from build123d import *

# Parameters (mm, degrees)
ESQUISSE1_R             = 22.5
BOSS_EXTRU_1_DEPTH      = 3
ESQUISSE2_R             = 5
BOSS_EXTRU_2_DEPTH      = 3
ENL_V_MAT_EXTRU_3_DEPTH = 10
ESQUISSE10_R            = 1.5
ENL_V_MAT_EXTRU_4_DEPTH = 10
ENL_V_MAT_EXTRU_5_DEPTH = 2.1
ESQUISSE12_R            = 0.515
ESQUISSE12_R_2          = 1.235
ENL_V_MAT_EXTRU_6_DEPTH = 33.057916339
ESQUISSE13_R            = 1.5
ENL_V_MAT_EXTRU_7_DEPTH = 33.380549717


with BuildPart() as part:
    # Esquisse1 → Boss.-Extru.1 (new body)
    with BuildSketch(Plane.XY):
        Circle(ESQUISSE1_R)
    extrude(amount=BOSS_EXTRU_1_DEPTH)

    # Esquisse2 → Boss.-Extru.2 (add)
    with BuildSketch(Plane.XY.offset(3)):
        Circle(ESQUISSE2_R)
    extrude(amount=BOSS_EXTRU_2_DEPTH)

    # Esquisse6 → Enlèv. mat.-Extru.3 (cut)
    with BuildSketch(Plane(origin=(0, 0, 0), x_dir=(-1, 0, 0), z_dir=(0, 0, -1))):
        with BuildLine():
            Line((-5, 19), (5, 19))
            ThreePointArc((5, 19), (6, 18), (5, 17))
            Line((5, 17), (-5, 17))
            ThreePointArc((-5, 17), (-6, 18), (-5, 19))
        make_face()
    extrude(amount=-ENL_V_MAT_EXTRU_3_DEPTH, mode=Mode.SUBTRACT)

    # Esquisse10 → Enlèv. mat.-Extru.4 (cut)
    with BuildSketch(Plane(origin=(0, 0, 0), x_dir=(-1, 0, 0), z_dir=(0, 0, -1))):
        with Locations((-9.835, -12)):
            Circle(ESQUISSE10_R)
        with Locations((9.831247904, -12)):
            Circle(ESQUISSE10_R)
    extrude(amount=-ENL_V_MAT_EXTRU_4_DEPTH, mode=Mode.SUBTRACT)

    # Esquisse11 → Enlèv. mat.-Extru.5 (cut)
    with BuildSketch(Plane.XY.offset(6)):
        with BuildLine():
            Line((2.516635816, 4.378246701), (2.643897714, 2.262786971))
            ThreePointArc((2.643897714, 2.262786971), (3.48, 0), (2.643897714, -2.262786971))
            Line((2.643897714, -2.262786971), (2.516635816, -4.378246701))
            ThreePointArc((2.516635816, -4.378246701), (0, -5.05), (-2.516635816, -4.378246701))
            Line((-2.516635816, -4.378246701), (-2.643897714, -2.262786971))
            ThreePointArc((-2.643897714, -2.262786971), (-3.48, 0), (-2.643897714, 2.262786971))
            Line((-2.643897714, 2.262786971), (-2.516635816, 4.378246701))
            ThreePointArc((-2.516635816, 4.378246701), (0, 5.05), (2.516635816, 4.378246701))
        make_face()
    extrude(amount=-ENL_V_MAT_EXTRU_5_DEPTH, mode=Mode.SUBTRACT)

    # Esquisse12 → Enlèv. mat.-Extru.6 (cut, through all)
    with BuildSketch(Plane.XY.offset(3.9)):
        with Locations((0, 4.25)):
            Circle(ESQUISSE12_R)
        Circle(ESQUISSE12_R_2)
        with Locations((0, -4.25)):
            Circle(ESQUISSE12_R)
    extrude(amount=-ENL_V_MAT_EXTRU_6_DEPTH, mode=Mode.SUBTRACT)

    # Esquisse13 → Enlèv. mat.-Extru.7 (cut, through all)
    with BuildSketch(Plane(origin=(0, 0, 0), x_dir=(-1, 0, 0), z_dir=(0, 0, -1))):
        with Locations((-9.835, 15.615)):
            Circle(ESQUISSE13_R)
        with Locations((9.831247904, 15.615)):
            Circle(ESQUISSE13_R)
    extrude(amount=-ENL_V_MAT_EXTRU_7_DEPTH, mode=Mode.SUBTRACT)


solid = part.part
Model file for the job. Use its own axes, mm. A direction names the side the tool comes from. Coordinates: 2 decimals unless noted, no trailing zeros. Loops run counter-clockwise (first coordinate to the right, second up) from the corner with the lowest first, then second, coordinate; pieces in that order, holes last. Notation, with made-up numbers: (6, -36) -> (41, -36) arc R16 ccw to (41, -6) -> close; hole circle Ø2 at (5, 75.25). An arc over 180 degrees is marked (long way). Use one line per item in the form item = value. Start each with the question number.
(1) Flat gauge pins, fed straight in: pin 1 (2 mm diameter, centred on x = -10, y = -2.5, fed in from +Z); pin 2 (1.5 mm diameter, centred on x = 2, z = 2, fed in from -Y); pin 3 (2.5 mm diameter, centred on x = 9.835, y = -12, fed in from +Z); pin 4 (1.6 mm diameter, centred on x = 0, y = -4.25, fed in from +Z). Where does each tip first touch, or does it go through?
(2) Cut at B-B on y = 0. Give the cut face in (x, z) (3 decimals).
(3) Cut at C-C on z = 1.8. Give the number of separate pieces and of enclosed holes in the cut face, and give its area (3 significant figures).
(4) Tool access for faces 1 (the flat face through (-4, 0, 6)), 2 (the flat face through (0, 19, 1)), 3 (the flat face through (2.583, -3.276, 4.965)): list every direction of +Z, -Z, +X, -X, +Y, -Y with a clear straight run to the whole face (end or side of a thin tool).
(5) Pull direction Y, two halves, no side cores. Call faces 4 (the flat face through (2.58, 3.3, 4.96)), 5 (the flat face through (0, -5, 0)), 6 (the cylindrical face through (-0.651, 4.957, 3.479)): pulls with the +Y half, pulls with the -Y half, needs draft (parallel to the pull), parting line crosses it, or undercut.
(6) Cut at D-D on y = -12. Give the cut face in (x, z) (3 decimals).
(7) Probe probe 1 along Y at (x, z) = (0, 2.2) (3 decimals); probe 2 along Z at (x, y) = (7, 17); probe 3 along X at (y, z) = (-4.5, 1.2). List the from-to ranges inside material, lowest first. Write a range as from..to.
(8) Cut at A-A on x = 0. Give the cut face in (y, z) (3 decimals), and give its area (3 significant figures).
Values:
q1.pin_1 = 3
q1.pin_2 = -22.47
q1.pin_3 = through
q1.pin_4 = 3.9
q2.outline = (-22.5, 0) -> (-1.235, 0) -> (-1.235, 3.9) -> (-3.48, 3.9) -> (-3.48, 6) -> (-5, 6) -> (-5, 3) -> (-22.5, 3) -> close; (1.235, 0) -> (22.5, 0) -> (22.5, 3) -> (5, 3) -> (5, 6) -> (3.48, 6) -> (3.48, 3.9) -> (1.235, 3.9) -> close
q3.separate_pieces = 1
q3.enclosed_holes = 8
q3.area = 1,530 mm2
q4.face_1 = +Z, +X, -X, +Y, -Y
q4.face_2 = +Z, -Z
q4.face_3 = +Z
q5.face_4 = undercut
q5.face_5 = needs draft
q5.face_6 = parting line crosses it
q6.outline = (-19.033, 0) -> (-11.331, 0) -> (-11.331, 3) -> (-19.033, 3) -> close; (-8.331, 0) -> (8.335, 0) -> (8.335, 3) -> (-8.331, 3) -> close; (11.335, 0) -> (19.033, 0) -> (19.033, 3) -> (11.335, 3) -> close
q7.probe_1 = -22.5..-4.765, -3.735..-1.235, 1.235..3.735, 4.765..17, 19..22.5
q7.probe_2 = 0..3
q7.probe_3 = -22.05..-0.45, 0.45..22.05
q8.outline = (-22.5, 0) -> (-4.765, 0) -> (-4.765, 3.9) -> (-5, 3.9) -> (-5, 3) -> (-22.5, 3) -> close; (-3.735, 0) -> (-1.235, 0) -> (-1.235, 3.9) -> (-3.735, 3.9) -> close; (1.235, 0) -> (3.735, 0) -> (3.735, 3.9) -> (1.235, 3.9) -> close; (4.765, 0) -> (17, 0) -> (17, 3) -> (5, 3) -> (5, 3.9) -> (4.765, 3.9) -> close; (19, 0) -> (22.5, 0) -> (22.5, 3) -> (19, 3) -> close
q8.area = 120 mm2
